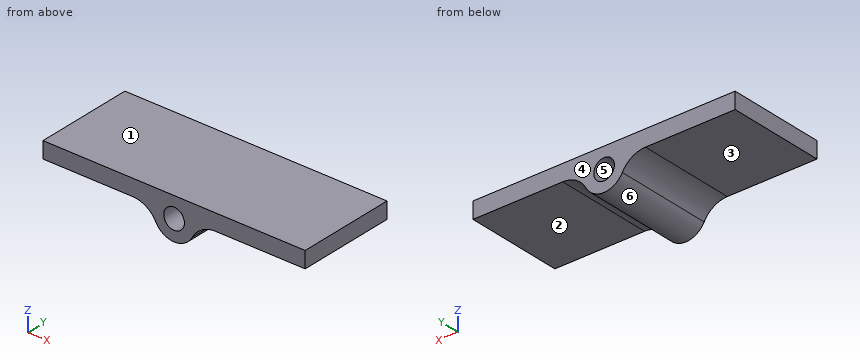
from build123d import *

# Parameters (mm, degrees)
SKETCH1_R           = 1
BOSS_EXTRUDE1_DEPTH = 9.525
FILLET1_R           = 2.54


with BuildPart() as part:
    # Sketch1 → Boss-Extrude1 (new body)
    with BuildSketch(Plane(origin=(0, 0, 0), x_dir=(1, 0, 0), z_dir=(0, 1, 0))):
        with BuildLine():
            Line((-12.7, -0.4125), (-12.7, -2))
            Line((-12.7, -2), (12.7, -2))
            Line((12.7, -2), (12.7, -0.4125))
            Line((12.7, -0.4125), (1.956998659, -0.4125))
            ThreePointArc((1.956998659, -0.4125), (0, 2), (-1.956998659, -0.4125))
            Line((-1.956998659, -0.4125), (-12.7, -0.4125))
        make_face()
        Circle(SKETCH1_R, mode=Mode.SUBTRACT)
    extrude(amount=BOSS_EXTRUDE1_DEPTH)

    # Fillet1
    fillet1_edges = [part.edges().sort_by_distance(p)[0] for p in [
        (-1.956998659, 4.7625, 0.4125),
        (1.956998659, 4.7625, 0.4125),
    ]]
    fillet(fillet1_edges, radius=FILLET1_R)


solid = part.part
Model file for the job. Use its own axes, mm. Face numbers are marked on the shaded views. A direction names the side the tool comes from. Give positions to 0.01 mm unless a question says otherwise; leave off trailing zeros. Order: outer loops, then holes, each group sorted by start corner. A loop starts at its lowest first (then second) coordinate and runs counter-clockwise, first axis right, second up. Notation, with made-up numbers: (12, -12.75) - (38, -12.75) arc R8 cw to (38, -8.75) - close; hole circle Ø9 at (42, 46.25). An arc over 180 degrees is marked (long way). Return JSON: item names as keys, results as strings.
1) Cut at D-D, the plane x = 7. Give the cut face in (y, z) (1 decimal).
Geometry says:
{"outline": "(0, 0.4) - (9.5, 0.4) - (9.5, 2) - (0, 2) - close"}
2) Pull direction X, two halves, no side cores. Call the marked faces 4, 5 and 6: pulls with the +X half, pulls with the -X half, needs draft (parallel to the pull), parting line crosses it, or undercut.
Geometry says:
{"face 4": "needs draft", "face 5": "undercut", "face 6": "parting line crosses it"}
3) Probe line 1 (Z direction, x = 0, y = 2.5); line 2 (Z direction, x = -10, y = 2); line 3 (X direction, y = 6, z = 0.9). List the from-to ranges inside material, lowest first. Write a range as from..to.
Geometry says:
{"line 1": "-2..-1, 1..2", "line 2": "0.41..2", "line 3": "-12.7..-0.44, 0.44..12.7"}
4) 3-axis set-ups, long thin cutter, end or side, ignore diameter. For the marked faces 1, 2 and 3: which of +Z, -Z, +X, -X, +Y, -Y reach the whole face in a straight line?
Geometry says:
{"face 1": "+Z, +X, -X, +Y, -Y", "face 2": "-Z, +X, +Y, -Y", "face 3": "-Z, -X, +Y, -Y"}
5) Cut at C-C, the plane z = 0.65. Give the cut face in (x, y) (3 decimals).
Geometry says:
{"outline": "(-12.7, 0) - (-0.76, 0) - (-0.76, 9.525) - (-12.7, 9.525) - close; (0.76, 0) - (12.7, 0) - (12.7, 9.525) - (0.76, 9.525) - close"}
6) Cut at B-B, the plane y = 1. Give the cut face in (x, z).
Geometry says:
{"outline": "(-12.7, 0.41) - (-4.01, 0.41) arc R2.54 cw to (-1.77, -0.94) arc R2 ccw to (1.77, -0.94) arc R2.54 cw to (4.01, 0.41) - (12.7, 0.41) - (12.7, 2) - (-12.7, 2) - close; hole circle Ø2 at (0, 0)"}
7) Cut at A-A, the plane x = 0. Give the cut face in (y, z) (3 decimals).
Geometry says:
{"outline": "(0, -2) - (9.525, -2) - (9.525, -1) - (0, -1) - close; (0, 1) - (9.525, 1) - (9.525, 2) - (0, 2) - close"}
8) Flat gauge pin, fed straight in: P1, Ø2.5, axis at x = -8, y = 4, coming from the -Z side. Where does the tip first touch, or does it go through?
Geometry says:
{"P1": "z = 0.41"}
